Answer from the drawing. Dimensions are ordinates in mm from the lowest x, y and z of the part. Coordinates: 2 decimals unless noted, no trailing zeros. Loops run counter-clockwise (first coordinate to the right, second up) from the corner with the lowest first, then second, coordinate; pieces in that order, holes last. Notation, with made-up numbers: M 65.25,14.5 L 75.25,14.5 A36 cw 75.25,48.5 Z; hole C -2,-8 d1. An arc over 180 degrees is marked long. Put each result on its own line as item: value.
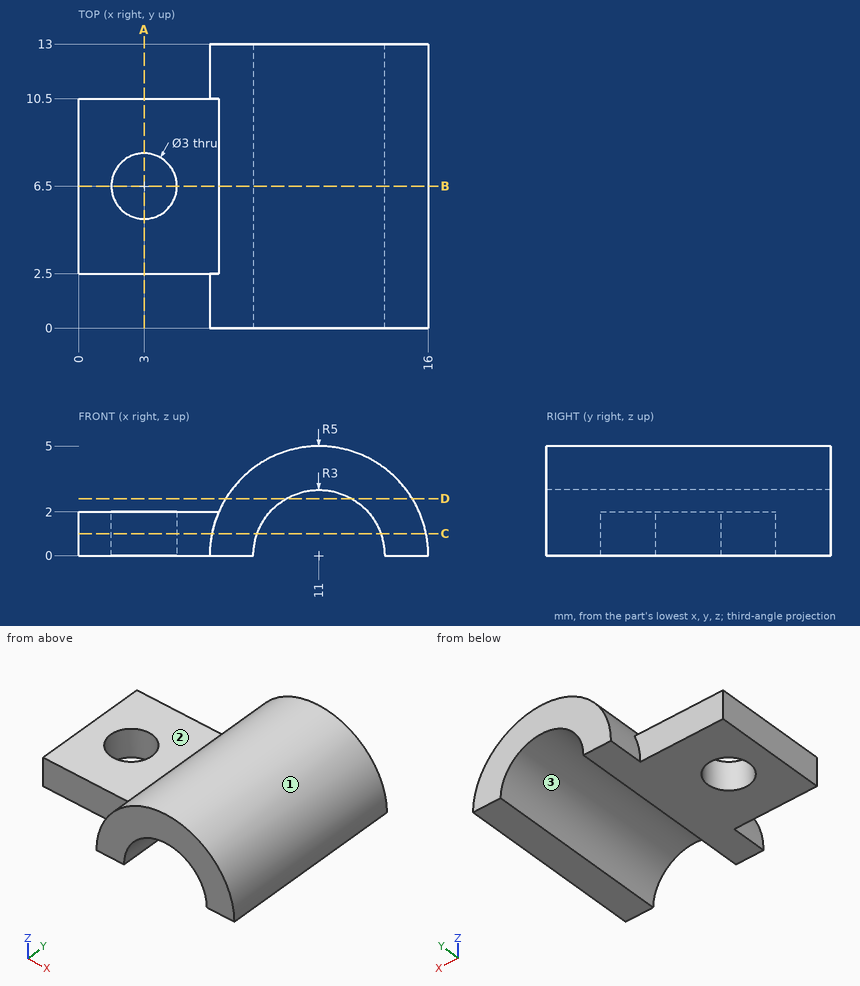
1) Given pin 1 Ø1 at (x, z) = (2, 1) entering from -Y; pin 2 Ø3 at (x, y) = (10.5, 6.5) entering from +Z; pin 3 Ø1 at (x, z) = (2, 1) entering from +Y; pin 4 Ø4 at (x, y) = (5, 6.5) entering from +Z, each flat-ended and moving along its own axis, determine where each tip first touches the part or whether it passes through.
Answer list:
pin 1: stops at y = 2.5
pin 2: stops at z = 5
pin 3: stops at y = 10.5
pin 4: stops at z = 3
2) Determine the mould class of the marked faces 1, 2 and 3 for opening direction X: released by +X, released by -X, zero draft, split by the parting line, or undercut.
Answer list:
face 1: split by the parting line
face 2: zero draft
face 3: undercut
3) Find section D-D, the plane z = 2.6. Write down the section's boundary in (x, y), plus the area to 3 significant figures.
Answer list:
outline: M 6.73,0 L 9.5,0 L 9.5,13 L 6.73,13 Z; M 12.5,0 L 15.27,0 L 15.27,13 L 12.5,13 Z
area: 72.1 mm^2
4) Find section A-A, the plane x = 3. Write down the section's boundary in (y, z), plus the area to 3 significant figures.
Answer list:
outline: M 2.5,0 L 5,0 L 5,2 L 2.5,2 Z; M 8,0 L 10.5,0 L 10.5,2 L 8,2 Z
area: 10.0 mm^2
5) Straight lines are drawn through the part: line 1 (Y direction, x = 3, z = 1.45); line 2 (X direction, y = 5.75, z = 0.35); line 3 (Z direction, x = 15, y = 10.25). For each, find the intervals that lie inside material, in ascending order. Write a range as [from, to].
Answer list:
line 1: y = [2.5, 5], [8, 10.5]
line 2: x = [0, 1.7], [4.3, 8.02], [13.98, 15.99]
line 3: z = [0, 3]
6) Find section C-C, the plane z = 1. Write down the section's boundary in (x, y).
Answer list:
outline: M 0,2.5 L 6.1,2.5 L 6.1,0 L 8.17,0 L 8.17,13 L 6.1,13 L 6.1,10.5 L 0,10.5 Z; M 13.83,0 L 15.9,0 L 15.9,13 L 13.83,13 Z; hole C 3,6.5 d3
7) Find section B-B, the plane y = 6.5. Write down the section's boundary in (x, z), plus the area to 3 significant figures.
Answer list:
outline: M 0,0 L 1.5,0 L 1.5,2 L 0,2 Z; M 4.5,0 L 8,0 A3 cw 14,0 L 16,0 A5 ccw 6.42,2 L 4.5,2 Z
area: 31.4 mm^2
